```python
from build123d import *

# Parameters (mm, degrees)
BOSS_EXTRUDE1_DEPTH = 6.35
CUT_EXTRUDE1_DEPTH  = 918.402376548
SKETCH3_R           = 52.07
CUT_EXTRUDE2_DEPTH  = 918.402376548


with BuildPart() as part:
    # Sketch1 → Boss-Extrude1 (new body)
    with BuildSketch(Plane(origin=(0, 0, 0), x_dir=(1, 0, 0), z_dir=(0, 1, 0))):
        with BuildLine():
            Line((-861.694916994, -269.761320345), (861.694916994, -269.761320345))
            add(Edge.make_bspline(
                [(861.694916994, -269.761320345), (876.821320345, -269.761320345), (876.821320345, -254.634916994)],
                knots=[5.505213485, 5.505213485, 5.505213485, 7.061157129, 7.061157129, 7.061157129], degree=2, weights=[1, 0.712338451, 1]))
            Line((876.821320345, -254.634916994), (876.821320345, 254.634916994))
            add(Edge.make_bspline(
                [(876.821320345, 254.634916994), (876.821320345, 269.761320345), (861.694916994, 269.761320345)],
                knots=[5.505213485, 5.505213485, 5.505213485, 7.061157129, 7.061157129, 7.061157129], degree=2, weights=[1, 0.712338451, 1]))
            Line((861.694916994, 269.761320345), (-861.694916994, 269.761320345))
            add(Edge.make_bspline(
                [(-861.694916994, 269.761320345), (-876.821320345, 269.761320345), (-876.821320345, 254.634916994)],
                knots=[5.505213485, 5.505213485, 5.505213485, 7.061157129, 7.061157129, 7.061157129], degree=2, weights=[1, 0.712338451, 1]))
            Line((-876.821320345, 254.634916994), (-876.821320345, -254.634916994))
            add(Edge.make_bspline(
                [(-876.821320345, -254.634916994), (-876.821320345, -269.761320345), (-861.694916994, -269.761320345)],
                knots=[5.505213485, 5.505213485, 5.505213485, 7.061157129, 7.061157129, 7.061157129], degree=2, weights=[1, 0.712338451, 1]))
        make_face()
    extrude(amount=BOSS_EXTRUDE1_DEPTH)

    # Sketch2 → Cut-Extrude1 (cut, through all)
    with BuildSketch(Plane(origin=(0, 6.35, 0), x_dir=(1, 0, 0), z_dir=(0, 1, 0))):
        with BuildLine():
            Line((-825.954313113, 134.591457199), (-767.566332113, 76.203476199))
            ThreePointArc((-767.566332113, 76.203476199), (-719.067867535, 56.114754417), (-670.569402958, 76.203476199))
            Line((-670.569402958, 76.203476199), (-612.181421958, 134.591457199))
            ThreePointArc((-612.181421958, 134.591457199), (-598.021653058, 171.575128433), (-616.092530237, 206.813380252))
            ThreePointArc((-616.092530237, 206.813380252), (-719.067867535, 243.07718636), (-822.043204833, 206.813380252))
            ThreePointArc((-822.043204833, 206.813380252), (-840.114082012, 171.575128433), (-825.954313113, 134.591457199))
        make_face()
    extrude(amount=-CUT_EXTRUDE1_DEPTH, mode=Mode.SUBTRACT)

    # Sketch3 → Cut-Extrude2 (cut, through all)
    with BuildSketch(Plane(origin=(0, 6.35, 0), x_dir=(1, 0, 0), z_dir=(0, 1, 0))):
        with Locations(Location((-754.506388348, -181.844577047, 0), (0, 0, 270))):
            Circle(SKETCH3_R)
    extrude(amount=-CUT_EXTRUDE2_DEPTH, mode=Mode.SUBTRACT)


solid = part.part
```
Source: CAD feature listing. Evaluate the final solid. Frame: model axes, mm. A direction names the side the tool comes from. Give positions to 0.01 mm unless a question says otherwise; leave off trailing zeros. Loops run counter-clockwise (first coordinate to the right, second up) from the corner with the lowest first, then second, coordinate; pieces in that order, holes last. Notation, with made-up numbers: (-10, -9) -> (6, -9) arc R23 ccw to (6, 7) -> close; hole circle Ø4 at (85, 86). An arc over 180 degrees is marked (long way). Use a Markdown table: item, result. Add a question column.
(1) Ray query, line 1 (Z direction, x = -707, y = 4.25); line 2 (Z direction, x = -656.5, y = 4.75); line 3 (X direction, y = 2.75, z = 160). Return the intervals inside material, ascending.
(2) Pull-direction query (X, two-part tool) for faces 1 (the face through (-12, 6.35, -4)), 2 (the face through (-717.51, 3.22, -243.07)); classes: +X half, -X half, draft (parallel to the pull), parting line (faces both ways), or undercut.
(3) Access query for faces 3 (the face through (-12, 0, -4)), 4 (the face through (-641.784, 3.219, -104.989)). Directions: +Z, -Z, +X, -X, +Y, -Y. A direction counts if a zero-diameter tool reaches every point of the face in a straight line with its end or side. Return the directions, or none.
(4) Section query C-C (y = 4.5). Count the separate pieces of the cut face and the enclosed holes in it, then the cut area to 3 significant figures.
(5) Section query B-B (z = -113). Output: boundary loops of the cut face in (x, y), then the cut area to 3 significant figures.
(6) Section query A-A (z = 189). Output: boundary loops of the cut face in (x, y), then the cut area to 3 significant figures.
Checked values:
| question | item | result |
|---|---|---|
| 1 | line 1 | -269.76 to -242.63, -57.18 to 160.53, 203.16 to 269.76 |
| 1 | line 2 | -269.76 to -230.7, -90.27 to 269.76 |
| 1 | line 3 | -876.82 to -801.77, -707.24 to 876.82 |
| 2 | face 1 | draft |
| 2 | face 2 | undercut |
| 3 | face 3 | +Z, -Z, +X, -X, -Y |
| 3 | face 4 | +Y, -Y |
| 4 | separate pieces | 1 |
| 4 | enclosed holes | 2 |
| 4 | area | 905,000 mm^2 |
| 5 | outline | (-876.82, 0) -> (-804.36, 0) -> (-804.36, 6.35) -> (-876.82, 6.35) -> close; (-633.77, 0) -> (876.82, 0) -> (876.82, 6.35) -> (-633.77, 6.35) -> close |
| 5 | area | 10,100 mm^2 |
| 6 | outline | (-876.82, 0) -> (-806.08, 0) -> (-806.08, 6.35) -> (-876.82, 6.35) -> close; (-702.93, 0) -> (876.82, 0) -> (876.82, 6.35) -> (-702.93, 6.35) -> close |
| 6 | area | 10,500 mm^2 |
